Here's how the part is built. I have some questions about the finished solid (model axes, mm). Face numbers are marked on the shaded views. A direction names the side the tool comes from. Coordinates: 2 decimals unless noted, no trailing zeros. Write each loop counter-clockwise with the first axis right and the second up, starting at its lowest first coordinate (ties: lowest second). Pieces come first, ordered by that corner, then holes. Notation, with made-up numbers: (64.5, 36) -> (95.5, 36) arc R9 cw to (95.5, 44) -> close; hole circle Ø5 at (79.5, 60). An arc over 180 degrees is marked (long way). Put each result on its own line as item: value. Start each with the question number.
Item 1: I want a section at D-D, the plane y = 62.5. List the corners of the cut face in (x, z) for me, then the cut area to 3 significant figures.
Item 2: On a 3-axis mill with a long thin cutter (end or side, diameter ignored), from which of +Z, -Z, +X, -X, +Y, -Y can I reach the whole of each face in a straight line? I mean the marked faces 1 and 2. Say none if no direction works.
Item 3: I want a section at C-C, the plane z = 27. List the corners of the cut face in (x, y) for me.
Item 4: I want a section at A-A, the plane y = 38. List the corners of the cut face in (x, z) for me, then the cut area to 3 significant figures.
Item 5: I want a section at B-B, the plane x = 49. List the corners of the cut face in (y, z) for me, then the cut area to 3 significant figures.
Item 6: For pin 1 (1.5 mm diameter, centred on x = 36.5, z = 35.5, fed in from -Y), with a flat end and sliding along its axis, tell me the tip position at first contact or that it passes through.
Item 7: If we mould it in two halves opening along Z, with no side actions, what happens to the marked faces 3, 4 and 5? For each: released by +Z, released by -Z, zero draft, split by the parting line, or undercut.
Item 8: I need wall thicknesses on line 1 (Z direction, x = -43.5, y = 21.5); line 2 (X direction, y = 43.5, z = 19.5); line 3 (Y direction, x = -40, z = 16.5). Which ranges of each line are inside material? Lowest first, please. Write a range as [from, to].
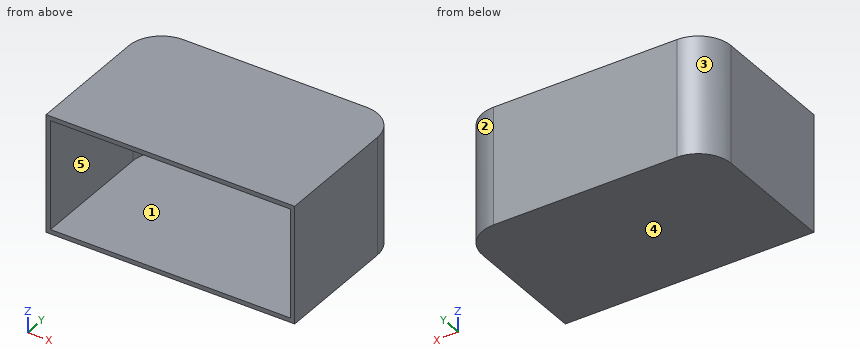
from build123d import *

# Parameters (mm, degrees)
F1_DEPTH = 54
F2_T     = -2


with BuildPart() as f1:
    # F0 (on Top) → F1 (new body)
    with BuildSketch(Plane.XY):
        with BuildLine():
            Line((-57, 57), (-57, 0))
            Line((-57, 0), (0, 0))
            Line((0, 0), (57, 0))
            Line((57, 0), (57, 57))
            ThreePointArc((57, 57), (52.606602, 67.606602), (42, 72))
            Line((42, 72), (0, 72))
            Line((0, 72), (-42, 72))
            ThreePointArc((-42, 72), (-52.606602, 67.606602), (-57, 57))
        make_face()
    extrude(amount=F1_DEPTH)

    # F2
    f2_openings = [f1.faces().sort_by_distance(p)[0] for p in [
        (0, 0, 27),
    ]]
    offset(amount=F2_T, openings=f2_openings)


solid = f1.part
Calculated:
1. outline: (-55.96, 0) -> (55.96, 0) -> (55.96, 54) -> (-55.96, 54) -> close; hole (-53.78, 2) -> (53.78, 2) -> (53.78, 52) -> (-53.78, 52) -> close
1. area: 665 mm2
2. face 1: -Y
2. face 2: +Z, -Z, +X, +Y
3. outline: (-57, 0) -> (-55, 0) -> (-55, 57) arc R13 cw to (-42, 70) -> (42, 70) arc R13 cw to (55, 57) -> (55, 0) -> (57, 0) -> (57, 57) arc R15 ccw to (42, 72) -> (-42, 72) arc R15 ccw to (-57, 57) -> close
4. outline: (-57, 0) -> (57, 0) -> (57, 54) -> (-57, 54) -> close; hole (-55, 2) -> (55, 2) -> (55, 52) -> (-55, 52) -> close
4. area: 656 mm2
5. outline: (0, 0) -> (70.27, 0) -> (70.27, 54) -> (0, 54) -> (0, 52) -> (67.95, 52) -> (67.95, 2) -> (0, 2) -> close
5. area: 397 mm2
6. pin 1: stops at y = 70
7. face 3: zero draft
7. face 4: released by -Z
7. face 5: undercut
8. line 1: z = [0, 2], [52, 54]
8. line 2: x = [-57, -55], [55, 57]
8. line 3: y = [70, 72]
